```python
from build123d import *

# Parameters (mm, degrees)
F0_R            = 38.1
F0_R_2          = 14.1605
F1_DEPTH        = 3.175
F2_R            = 2.3622
F3_DEPTH        = 3.176
F3_COPIES_COUNT = 6


# Not quite as in the source:
# - a pattern or mirror of a feature is missing from the dataset's text; its kind, count and spacing are read off the source's solid


with BuildPart() as f1:
    # F0 (on Top) → F1 (new body)
    with BuildSketch(Plane.XY):
        Circle(F0_R)
        Circle(F0_R_2, mode=Mode.SUBTRACT)
    extrude(amount=F1_DEPTH)

    # F2 (on face) → F3 (cut, through all)
    with BuildSketch(Plane.XY.offset(3.175)):
        with Locations((0, 23.8125)):
            Circle(F2_R)
    f3 = extrude(amount=-F3_DEPTH, mode=Mode.SUBTRACT)

    # F3_copies: F3 ×6 about axis
    f3_copies_axis = Axis((0, 0, 0), (0, 0, 1))
    for i in range(1, F3_COPIES_COUNT):
        add(f3.rotate(f3_copies_axis, i * 360 / F3_COPIES_COUNT), mode=Mode.SUBTRACT)


solid = f1.part
```
Check sheet for the modelled part. Datum: model origin and axes. Units: mm. Round coordinates to 2 decimals unless told otherwise and drop trailing zeros. Order: outer loops, then holes, each group sorted by start corner. A loop starts at its lowest first (then second) coordinate and runs counter-clockwise, first axis right, second up.
1) Section check D-D (x = 11). Record the boundary of the cut face in (y, z) (3 decimals), and give its area (3 significant figures).
2) Section check C-C (z = 1.15). Record the boundary of the cut face in (x, y).
3) Section check A-A (x = 0). Record the boundary of the cut face in (y, z) (1 decimal), and give its area (3 significant figures).
4) Mould release check, pull along X, two halves, no side actions. Record for faces 1 (the flat face through (16, 1, 0)), 2 (the cylindrical face through (-30.235, -23.183, 1.565)), 3 (the cylindrical face through (18.37, 11.2, 1.61)), 4 (the cylindrical face through (-22.875, 11.197, 1.61)): +X half, -X half, draft (parallel to the pull), parting line (faces both ways), or undercut.
5) Section check B-B (y = 0). Record the boundary of the cut face in (x, z) (1 decimal).
6) Scan lines: line 1 (Y direction, x = 0, z = 0.85); line 2 (Y direction, x = -21.5, z = 0.4); line 3 (Y direction, x = -18.5, z = 2.4). Record each from-to range of solid material in increasing order.
7) Go/stop test with flat-tipped pins: pin 1 Ø1 at (x, z) = (7, 1.5) entering from +Y; pin 2 Ø1 at (x, z) = (18.5, 0.5) entering from +Y. Record where each tip stops, or that it passes through.
Result:
1. outline: (-36.478, 0) - (-8.917, 0) - (-8.917, 3.175) - (-36.478, 3.175) - close; (8.917, 0) - (36.478, 0) - (36.478, 3.175) - (8.917, 3.175) - close
1. area: 175 mm2
2. outline: circle Ø76.2 at (0, 0); hole circle Ø4.72 at (-20.62, -11.91); hole circle Ø4.72 at (-20.62, 11.91); hole circle Ø28.32 at (0, 0); hole circle Ø4.72 at (0, -23.81); hole circle Ø4.72 at (0, 23.81); hole circle Ø4.72 at (20.62, -11.91); hole circle Ø4.72 at (20.62, 11.91)
3. outline: (-38.1, 0) - (-26.2, 0) - (-26.2, 3.2) - (-38.1, 3.2) - close; (-21.5, 0) - (-14.2, 0) - (-14.2, 3.2) - (-21.5, 3.2) - close; (14.2, 0) - (21.5, 0) - (21.5, 3.2) - (14.2, 3.2) - close; (26.2, 0) - (38.1, 0) - (38.1, 3.2) - (26.2, 3.2) - close
3. area: 122 mm2
4. face 1: draft
4. face 2: parting line
4. face 3: undercut
4. face 4: undercut
5. outline: (-38.1, 0) - (-14.2, 0) - (-14.2, 3.2) - (-38.1, 3.2) - close; (14.2, 0) - (38.1, 0) - (38.1, 3.2) - (14.2, 3.2) - close
6. line 1: y = -38.1 to -26.17, -21.45 to -14.16, 14.16 to 21.45, 26.17 to 38.1
6. line 2: y = -31.45 to -14.1, -9.71 to 9.71, 14.1 to 31.45
6. line 3: y = -33.31 to -12.94, -10.87 to 10.87, 12.94 to 33.31
7. pin 1: stops at y = 37.54
7. pin 2: stops at y = 33.58
